For this review, take the finished solid that the model builds, in its own axes (mm). Face numbers are marked on the shaded views. A direction names the side the tool comes from. Coordinates: 2 decimals unless noted, no trailing zeros. Loops run counter-clockwise (first coordinate to the right, second up) from the corner with the lowest first, then second, coordinate; pieces in that order, holes last. Notation, with made-up numbers: (57, 88) - (81, 88) arc R26 cw to (81, 114) - close; hole circle Ø9 at (89.5, 13.25). An arc over 180 degrees is marked (long way). Use one line per item in the form item = value. Start each with the question number.
1. Add section C-C on z = 21. Give the boundary of the cut face in (x, y), and give its area (3 significant figures).
2. Add section A-A on y = 0. Give the boundary of the cut face in (x, z), and give its area (3 significant figures).
3. To check wall thickness, follow probe 1 along X at (y, z) = (3, 26); probe 2 along Z at (x, y) = (3.75, -2.25). State the ranges of each line that lie inside material, in increasing order.
4. Machinability: for the marked faces 1 and 2, which of the approach directions +Z, -Z, +X, -X, +Y, -Y give a long, thin tool a straight path to every point of the face, cutting with its end or side? Answer none if there is none.
5. Add section D-D on z = 36. Give the boundary of the cut face in (x, y), and give its area (3 significant figures).
6. For pin 1 Ø1 at (x, z) = (-4, 28.5) entering from +Y; pin 2 Ø3 at (x, y) = (1, -4) entering from -Z; pin 3 Ø3 at (x, z) = (-3, 26.5) entering from -Y; pin 4 Ø3 at (x, z) = (-3, 36) entering from -Y, all flat-tipped, find the tip position at first contact; note any pin that passes through.
```python
from build123d import *

# Parameters (mm, degrees)
ESQUISSE1_R          = 5
BASE_EXTRUSION_DEPTH = 35
ESQUISSE4_R          = 4
BOSS_EXTRU_1_DEPTH   = 8
CHANFREIN1_SIZE      = 0.8


with BuildPart() as part:
    # Esquisse1 → Base-Extrusion (new body)
    with BuildSketch(Plane.XY):
        Circle(ESQUISSE1_R)
    extrude(amount=BASE_EXTRUSION_DEPTH)

    # Esquisse4 → Boss.-Extru.1 (add)
    with BuildSketch(Plane.XY.offset(35)):
        Circle(ESQUISSE4_R)
    extrude(amount=BOSS_EXTRU_1_DEPTH)

    # Chanfrein1
    chanfrein1_edges = [part.edges().sort_by_distance(p)[0] for p in [
        (-4, 0, 43),
    ]]
    chamfer(chanfrein1_edges, length=CHANFREIN1_SIZE)


solid = part.part
```
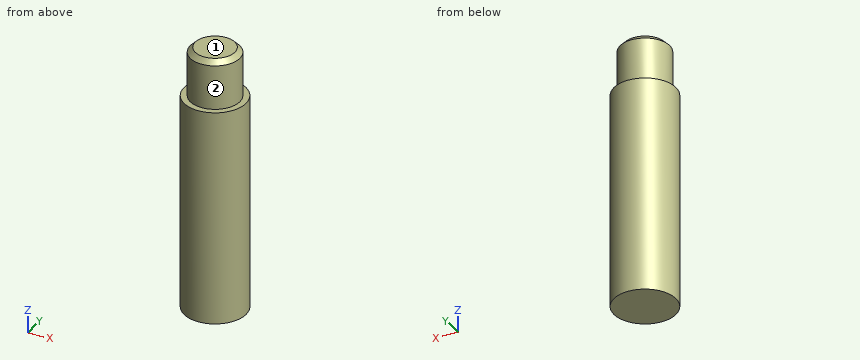
Conclusion:
q1.outline = circle Ø10 at (0, 0)
q1.area = 78.5 mm^2
q2.outline = (-5, 0) - (5, 0) - (5, 35) - (4, 35) - (4, 42.2) - (3.2, 43) - (-3.2, 43) - (-4, 42.2) - (-4, 35) - (-5, 35) - close
q2.area = 413 mm^2
q3.probe_1 = -4 to 4
q3.probe_2 = 0 to 35
q4.face_1 = +Z, +X, -X, +Y, -Y
q4.face_2 = +Z
q5.outline = circle Ø8 at (0, 0)
q5.area = 50.3 mm^2
q6.pin_1 = 3.57
q6.pin_2 = 0
q6.pin_3 = -4.77
q6.pin_4 = -4.63
